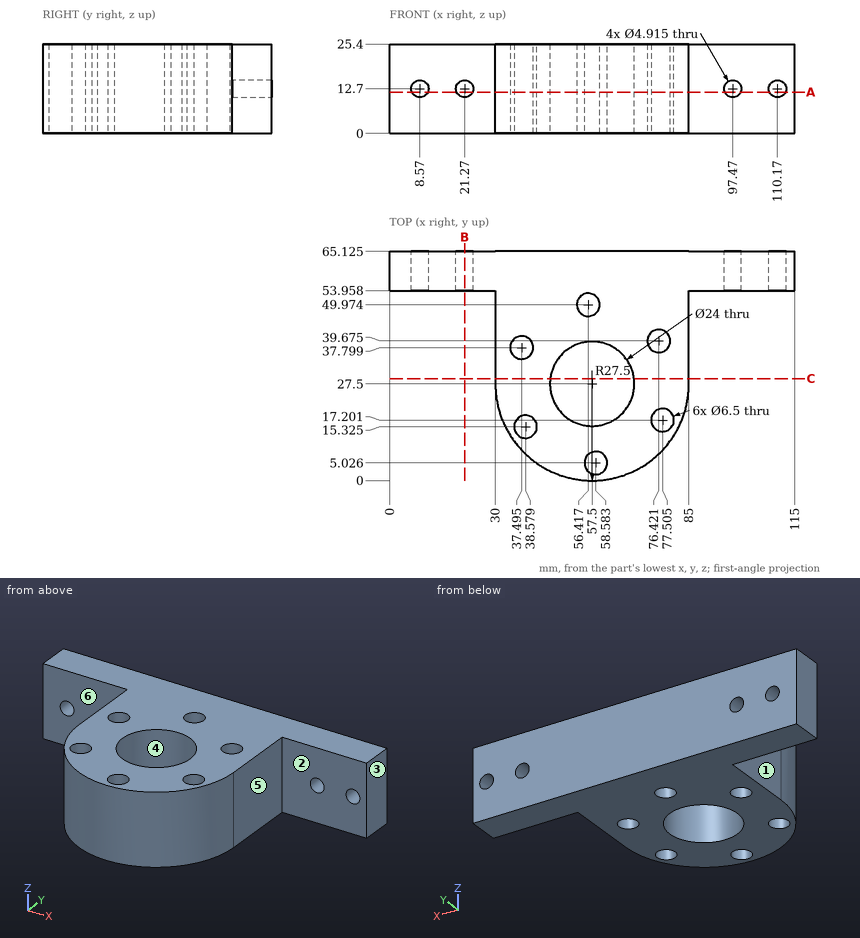
For this review, use the dimensioned drawing (mm, ordinates from the lowest corner) and the shaded views. A direction names the side the tool comes from. Round coordinates to 2 decimals unless told otherwise and drop trailing zeros. Order: outer loops, then holes, each group sorted by start corner. A loop starts at its lowest first (then second) coordinate and runs counter-clockwise, first axis right, second up. Notation, with made-up numbers: (82, -35) - (108, -35) arc R33 cw to (108, 4) - close; hole circle Ø4 at (-40, 74). An arc over 180 degrees is marked (long way). Use one line per item in the form item = value.
Q1. Add section A-A on z = 11.75. Give the number of separate pieces and of enclosed holes in the cut face, then the cut area to 3 significant figures.
Response values:
separate_pieces = 5
enclosed_holes = 7
area = 3,070 mm^2
Q2. Clearance check with flat-ended pins moving along their axes: P1, Ø4, axis at x = 102.5, z = 22.5, coming from the -Y side; P2, Ø1.5, axis at y = 29, z = 13.5, coming from the -X side; P3, Ø8, axis at y = 21.5, z = 21, coming from the -X side. State where each tip first meets the part, or that it passes through.
Response values:
P1 = 53.96
P2 = 30
P3 = 30.07
Q3. Tool access review of the marked faces 1, 2 and 3: name each direction out of +Z, -Z, +X, -X, +Y, -Y from which nothing blocks a thin tool from reaching the whole face with its end or side.
Response values:
face_1 = +Z, -Z, -X, -Y
face_2 = +Z, -Z, +X, -Y
face_3 = +Z, -Z, +X, +Y, -Y
Q4. Add section C-C on y = 29. Give the boundary of the cut face in (x, z) (1 decimal), then the cut area to 3 significant figures.
Response values:
outline = (30, 0) - (45.6, 0) - (45.6, 25.4) - (30, 25.4) - close; (69.4, 0) - (85, 0) - (85, 25.4) - (69.4, 25.4) - close
area = 792 mm^2
Q5. Mouldability with a two-part tool opening along Y and no side actions: class the marked faces 4, 5 and 6 as pulls with the +Y half, pulls with the -Y half, needs draft (parallel to the pull), parting line crosses it, or undercut.
Response values:
face_4 = undercut
face_5 = needs draft
face_6 = pulls with the -Y half
Q6. Add section B-B on x = 21.27. Give the boundary of the cut face in (y, z) (1 decimal).
Response values:
outline = (54, 0) - (65.1, 0) - (65.1, 10.2) - (54, 10.2) - close; (54, 15.2) - (65.1, 15.2) - (65.1, 25.4) - (54, 25.4) - close
Q7. To check wall thickness, follow line 1 (X direction, y = 58.5, z = 12.7); line 2 (X direction, y = 40.5, z = 17.5) (1 decimal); line 3 (Y direction, x = 25.5, z = 2.25) (1 decimal). State the ranges of each line that lie inside material, in increasing order.
Response values:
line_1 = 0 to 6.11, 11.03 to 18.81, 23.73 to 95.01, 99.93 to 107.71, 112.63 to 115
line_2 = 30 to 35.7, 39.3 to 73.3, 79.6 to 85
line_3 = 54 to 65.1
